Can you work these out from the model? Positions are in its coordinate system, mm. Face numbers are marked on the shaded views. A direction names the side the tool comes from. Give positions to 0.01 mm unless a question says otherwise; leave off trailing zeros. Loops run counter-clockwise (first coordinate to the right, second up) from the corner with the lowest first, then second, coordinate; pieces in that order, holes last. Notation, with made-up numbers: M 54.5,-40 L 107.5,-40 A21 cw 107.5,-27 Z; hole C 80.25,57 d5. An arc over 180 degrees is marked long. Put each result on its own line as item: value. Start each with the question number.
1) For P1, Ø1.5, axis at x = 3, z = 4, coming from the +Y side, with a flat end and sliding along its axis, tell me the tip position at first contact or that it passes through.
2) Imagine slicing it at B-B (z = 3.5). Write out the boundary of the cut face in (x, y), then the cut area to 3 significant figures.
3) Please list where these lines run through material, in increasing order: line 1 along Y through (x, z) = (4.7, 4.45); line 2 along Y through (x, z) = (2.7, 3.1); line 3 along X through (y, z) = (-1.25, 3.7). Write a range as from..to.
4) Imagine slicing it at A-A (x = 3.5). Write out the boundary of the cut face in (y, z).
5) For the marked faces 1 and 2, which set-ups out of +Z, -Z, +X, -X, +Y, -Y let a thin tool reach every point of the face, with its end or its side?
from build123d import *

# Parameters (mm, degrees)
AUFSATZ_LINEAR_AUSTRAGEN1_OUTLINE_W = 3.1
AUFSATZ_LINEAR_AUSTRAGEN1_OUTLINE_H = 3.1
AUFSATZ_LINEAR_AUSTRAGEN1_DEPTH     = 15.5
SKIZZE2_R                           = 1.25
AUFSATZ_LINEAR_AUSTRAGEN2_DEPTH     = 1.8
FASE1_SIZE                          = 0.4


# Read off the part's stored shape, not the designer's step: Aufsatz-Linear austragen1
with BuildPart() as part:
    # Aufsatz-Linear austragen1 outline → Aufsatz-Linear austragen1 (new body)
    with BuildSketch(Plane(origin=(0, -17.3, 0), x_dir=(1, 0, 0), z_dir=(0, 1, 0))):
        with Locations((3.5, -3.5)):
            Rectangle(AUFSATZ_LINEAR_AUSTRAGEN1_OUTLINE_W, AUFSATZ_LINEAR_AUSTRAGEN1_OUTLINE_H)
    extrude(amount=AUFSATZ_LINEAR_AUSTRAGEN1_DEPTH)

    # Skizze2 → Aufsatz-Linear austragen2 (add)
    with BuildSketch(Plane(origin=(0, -1.8, 0), x_dir=(1, 0, 0), z_dir=(0, 1, 0))):
        with Locations(Location((3.5, -3.5, 0), (0, 0, 270))):
            Circle(SKIZZE2_R)
    extrude(amount=AUFSATZ_LINEAR_AUSTRAGEN2_DEPTH)

    # Fase1
    fase1_edges = [part.edges().sort_by_distance(p)[0] for p in [
        (3.5, 0, 2.25),
    ]]
    chamfer(fase1_edges, length=FASE1_SIZE)


solid = part.part
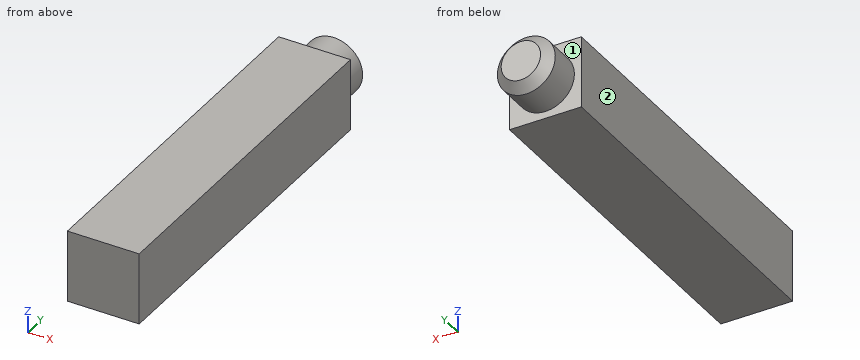
Recorded:
1. P1: y = 0
2. outline: M 1.95,-17.3 L 5.05,-17.3 L 5.05,-1.8 L 4.75,-1.8 L 4.75,-0.4 L 4.35,0 L 2.65,0 L 2.25,-0.4 L 2.25,-1.8 L 1.95,-1.8 Z
2. area: 52.4 mm²
3. line 1: -17.3..-1.8
3. line 2: -17.3..-0.04
3. line 3: 2.27..4.73
4. outline: M -17.3,1.95 L -1.8,1.95 L -1.8,2.25 L -0.4,2.25 L 0,2.65 L 0,4.35 L -0.4,4.75 L -1.8,4.75 L -1.8,5.05 L -17.3,5.05 Z
5. face 1: +Y
5. face 2: +Z, -Z, -X, +Y, -Y
